Work out the finished part from the listing and answer in its coordinate system (mm). Face numbers are marked on the shaded views. A direction names the side the tool comes from. Round coordinates to 2 decimals unless told otherwise and drop trailing zeros. Order: outer loops, then holes, each group sorted by start corner. A loop starts at its lowest first (then second) coordinate and runs counter-clockwise, first axis right, second up. Notation, with made-up numbers: (37, -33.5) - (96, -33.5) arc R31 cw to (96, 4.5) - close; hole circle Ø4 at (-31, 47). An arc over 180 degrees is marked (long way). One line per question, with ' | ' between items. Start each with the question number.
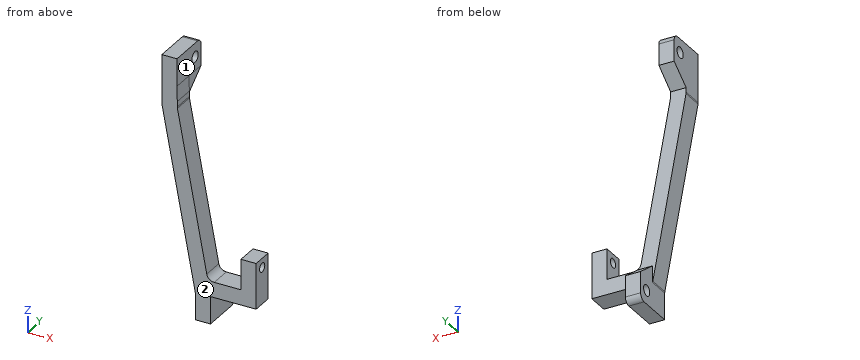
from build123d import *

# Parameters (mm, degrees)
BOSS_EXTRUDE1_DEPTH      = 7
BOSS_EXTRUDE2_START      = 7
SKETCH1_3_W              = 5
SKETCH1_3_H              = 9
BOSS_EXTRUDE2_DEPTH      = 7
M3_CLEARANCE_HOLE1_D     = 3.6
FILLET2_R                = 2.5
BOSS_EXTRUDE3_DEPTH      = 10
BOSS_EXTRUDE3_DEPTH_BACK = 5
SKETCH6_W                = 5
SKETCH6_H                = 7
SKETCH7_R                = 1.5
CUT_EXTRUDE1_DEPTH       = 10
FILLET6_R                = 2
SKETCH8_W                = 84
SKETCH8_H                = 14
CUT_EXTRUDE2_DEPTH       = 83.35289916
CHAMFER2_SIZE            = 7
CHAMFER2_SIZE_2          = 5.274878351


with BuildPart() as part:
    # Sketch1 → Boss-Extrude1 (new body)
    with BuildSketch(Plane(origin=(0, 0, 0), x_dir=(1, 0, 0), z_dir=(0, 1, 0))):
        Polygon((-23.5, -9), (-23.5, 0), (-23.413842004, 5), (-23.413842004, 7), (-13.346045394, 61), (13.346045394, 61), (23.413842004, 7), (23.413842004, 5), (23.5, 0), (23.5, -9), (28.5, -9), (28.5, 7), (17.5, 66), (17.5, 75), (12.5, 75), (12.5, 66), (-12.5, 66), (-12.5, 75), (-17.5, 75), (-17.5, 66), (-28.5, 7), (-28.5, -9), align=None)
    extrude(amount=BOSS_EXTRUDE1_DEPTH)

    # Sketch1<3> → Boss-Extrude2 (add)
    with BuildSketch(Plane(origin=(0, 0, 0), x_dir=(1, 0, 0), z_dir=(0, 1, 0)).offset(BOSS_EXTRUDE2_START)):
        with Locations((-15, 70.5)):
            Rectangle(SKETCH1_3_W, SKETCH1_3_H)
        with Locations((15, 70.5)):
            Rectangle(SKETCH1_3_W, SKETCH1_3_H)
        with Locations((-26, -4.5)):
            Rectangle(SKETCH1_3_W, SKETCH1_3_H)
        with Locations((26, -4.5)):
            Rectangle(SKETCH1_3_W, SKETCH1_3_H)
    extrude(amount=BOSS_EXTRUDE2_DEPTH)

    # M3 Clearance Hole1 (through all)
    with Locations(Plane(origin=(28.5, 0, 0), x_dir=(0, 0, -1), z_dir=(1, 0, 0))):
        with Locations((-4.5, 10.5), (70.5, 10.5)):
            Hole(M3_CLEARANCE_HOLE1_D / 2)

    # Fillet2
    fillet2_edges = [part.edges().sort_by_distance(p)[0] for p in [
        (-28.5, 3.5, -7),
        (-17.5, 3.5, -66),
        (17.5, 3.5, -66),
        (28.5, 3.5, -7),
        (23.413842004, 3.5, -5),
        (23.413842004, 3.5, -7),
        (13.346045394, 3.5, -61),
        (-13.346045394, 3.5, -61),
        (-23.413842004, 3.5, -7),
        (-23.413842004, 3.5, -5),
    ]]
    fillet(fillet2_edges, radius=FILLET2_R)

    # Sketch6 → Boss-Extrude3 (add, two sides: drawn at the far end of the back side and taken through both)
    with BuildSketch(Plane.XY.offset(-61).offset(-BOSS_EXTRUDE3_DEPTH_BACK)):
        with Locations((0, 3.5)):
            Rectangle(SKETCH6_W, SKETCH6_H)
    extrude(amount=BOSS_EXTRUDE3_DEPTH + BOSS_EXTRUDE3_DEPTH_BACK)

    # Sketch7 → Cut-Extrude1 (cut)
    with BuildSketch(Plane.ZY.offset(2.5)):
        with Locations(Location((-54, 3.5, 0), (0, 0, 270))):
            Circle(SKETCH7_R)
    extrude(amount=-CUT_EXTRUDE1_DEPTH, mode=Mode.SUBTRACT)

    # Fillet6
    fillet6_edges = [part.edges().sort_by_distance(p)[0] for p in [
        (26, 14, 9),
        (-15, 14, -75),
        (15, 14, -75),
        (-26, 14, 9),
    ]]
    fillet(fillet6_edges, radius=FILLET6_R)

    # Sketch8 → Cut-Extrude2 (cut, through all)
    with BuildSketch(Plane(origin=(2.5, 0, 0), x_dir=(0, 0, -1), z_dir=(1, 0, 0))):
        with Locations((33, 7)):
            Rectangle(SKETCH8_W, SKETCH8_H)
    extrude(amount=CUT_EXTRUDE2_DEPTH, mode=Mode.SUBTRACT)

    # Chamfer2
    # the kernel refuses this chamfer: 7, 5.274878351 mm, written as the material it adds along each edge
    with BuildSketch(Plane(origin=(-5.436042239, 7, 0), x_dir=(0, 0.9997280272590686, 0.023321052992758308), z_dir=(-1, 0, 0))) as chamfer2_piece_1_section:
        Polygon((CHAMFER2_SIZE * 0.999728027259, CHAMFER2_SIZE * 0.0233210529928), (-CHAMFER2_SIZE_2 * 0.0233210529915, CHAMFER2_SIZE_2 * 0.999728027206), (0, 0), align=None)
    chamfer2_piece_1 = extrude(amount=23.063957761, mode=Mode.PRIVATE)
    chamfer2_piece_1 = split(chamfer2_piece_1, bisect_by=Plane(origin=(-23.413842004, 8.750234769, -2.637085353), z_dir=(-1, 0, 0)), keep=Keep.TOP, mode=Mode.PRIVATE)
    chamfer2_piece_1 = split(chamfer2_piece_1, bisect_by=Plane(origin=(-23.454565548, 8.750234769, -2.636693852), z_dir=(-0.999851569048757, 0, -0.01722904149216463)), keep=Keep.TOP, mode=Mode.PRIVATE)
    add(chamfer2_piece_1)
    with BuildSketch(Plane(origin=(-17.5, 7, -66), x_dir=(2.839775720480132e-15, -0.0410460451010975, 0.9991572559820394), z_dir=(1, 0, 0))) as chamfer2_piece_2:
        Polygon((CHAMFER2_SIZE_2 * 0.999157255929, -CHAMFER2_SIZE_2 * 0.0410460450989), (-CHAMFER2_SIZE * 0.0410460451011, -CHAMFER2_SIZE * 0.999157255982), (0, 0), align=None)
    extrude(amount=5)


solid = part.part
1) Flat-ended cylindrical pins translate along their axes: pin 1 (2.5 mm diameter, centred on y = 7.5, z = 6.5, fed in from +X); pin 2 (3 mm diameter, centred on y = 10.5, z = -70.5, fed in from +X); pin 3 (7 mm diameter, centred on y = 9.5, z = -66.5, fed in from +X); pin 4 (5 mm diameter, centred on x = -9, y = 7, fed in from +Z). Find the tip coordinate at first contact, or state that the pin passes through.
2) Section D-D on x = -6 is taken. Give the vertices of the cut face in (y, z).
3) Section A-A on y = 3.5 is taken. Give the vertices of the cut face in (x, z), and give its area (3 significant figures).
4) Section B-B on z = -70.5 is taken. Give the vertices of the cut face in (x, y), and give its area (3 significant figures).
5) For the marked faces 1 and 2, determine the directions among +Z, -Z, +X, -X, +Y, -Y from which every point of the face is accessible in a straight line to the end or side of a thin tool.
6) Straight lines are drawn through the part: line 1 (Y direction, x = -24.75, z = 4.5); line 2 (X direction, y = 2.75, z = 0); line 3 (Y direction, x = -15, z = -61). For each, find the intervals that lie inside material, in ascending order.
7) Section C-C on z = -54 is taken. Give the vertices of the cut face in (x, y), and give its area (3 significant figures).
Recorded:
1) pin 1: stops at x = -23.5 | pin 2: passes through | pin 3: stops at x = 2.5 | pin 4: stops at z = -60.99
2) outline: (0, -66) - (7, -66) - (7, -61) - (0, -61) - close
3) outline: (-28.5, -6.77) arc R2.5 ccw to (-28.46, -7.23) - (-17.54, -65.77) arc R2.5 cw to (-17.5, -66.23) - (-17.5, -75) - (-12.5, -75) - (-12.5, -66) - (2.5, -66) - (2.5, -55.5) - (-2.5, -55.5) - (-2.5, -61) - (-11.27, -61) arc R2.5 cw to (-13.73, -58.96) - (-23.37, -7.23) arc R2.5 cw to (-23.41, -6.77) - (-23.41, -5) - (-23.5, 0) - (-23.5, 9) - (-28.5, 9) - close; (-2.5, -52.5) - (2.5, -52.5) - (2.5, -51) - (-2.5, -51) - close | area: 538 mm²
4) outline: (-17.5, 0) - (-12.5, 0) - (-12.5, 8.7) - (-17.5, 8.7) - close; (-17.5, 12.3) - (-12.5, 12.3) - (-12.5, 14) - (-17.5, 14) - close | area: 52.0 mm²
5) face 1: +Z, +X, +Y, -Y | face 2: +Z, -Z, +X, -X, -Y
6) line 1: y = 0 to 8.7, 12.3 to 14 | line 2: x = -28.5 to -23.5 | line 3: y = 0 to 7.36
7) outline: (-19.74, 0) - (-14.65, 0) - (-14.65, 7) - (-19.74, 7) - close; (-2.5, 0) - (2.5, 0) - (2.5, 2) - (-2.5, 2) - close; (-2.5, 5) - (2.5, 5) - (2.5, 7) - (-2.5, 7) - close | area: 55.6 mm²
